```python
from build123d import *

# Parameters (mm, degrees)
IZIM1_R                     = 2.5
Y_KSEKLIK_EKSTR_ZYON1_DEPTH = 6
IZIM5_R                     = 0.246458924
IZIM7_R                     = 0.245


with BuildPart() as part:
    # Çizim1 → Yükseklik-Ekstrüzyon1 (new body)
    with BuildSketch(Plane(origin=(0, 0, 0), x_dir=(0, 0, -1), z_dir=(1, 0, 0))):
        Circle(IZIM1_R)
    extrude(amount=Y_KSEKLIK_EKSTR_ZYON1_DEPTH)

    # Süpür1: sweep along a path in Çizim4
    with BuildLine(Plane.XY) as s_p_r1_path:
        Line((0, 0), (-2.33257059, 0))
        ThreePointArc((-2.33257059, 0), (-2.732509931, -0.165660299), (-2.89817023, -0.56559964))
        Line((-2.89817023, -0.56559964), (-2.89817023, -8.872558098))
    # Çizim5 → Süpür1 (sweep)
    with BuildSketch(Plane(origin=(-2.89817023, -8.872558098, 0), x_dir=(-1, 0, 0), z_dir=(0, -1, 0))):
        with Locations((-0.000978554, 0)):
            Circle(IZIM5_R)
    sweep(path=s_p_r1_path.line)

    # Süpür2: sweep along a path in Çizim6
    with BuildLine(Plane.XY) as s_p_r2_path:
        Line((6, 0), (8.33, 0))
        ThreePointArc((8.33, 0), (8.931040764, -0.248959236), (9.18, -0.85))
        Line((9.18, -0.85), (9.18, -9.16))
    # Çizim7 → Süpür2 (sweep)
    with BuildSketch(Plane(origin=(9.18, -9.16, 0), x_dir=(-1, 0, 0), z_dir=(0, -1, 0))):
        with Locations((-0.002407495, 0)):
            Circle(IZIM7_R)
    sweep(path=s_p_r2_path.line)


solid = part.part
```
Geometry: final body of the model. Coordinates: model frame, mm. Round coordinates to 2 decimals unless told otherwise and drop trailing zeros. Write each loop counter-clockwise with the first axis right and the second up, starting at its lowest first coordinate (ties: lowest second). Pieces come first, ordered by that corner, then holes.
Item 1: Pin query (flat end, axial travel): P1, Ø2, axis at y = -3.5, z = 2, coming from the +X side. Return the tip coordinate at first contact, or that it passes through.
Item 2: Material intervals for L1, parallel to X at y = 1, z = 2.1; L2, parallel to Y at x = -0.5, z = 0; L3, parallel to Y at x = 3, z = 0.2, sorted ascending.
Item 3: Section query C-C (y = -3.5). Return loops of the section in (x, z) (3 decimals), plus the area to 3 significant figures.
Item 4: Section query D-D (x = -1). Return loops of the section in (y, z).
Item 5: Section query A-A (y = -2). Return loops of the section in (x, z) (3 decimals).
Item 6: Section query B-B (z = 0). Return loops of the section in (x, y), plus the area to 3 significant figures.
Completed:
1. P1: passes through
2. L1: x = 0 to 6
2. L2: y = -0.25 to 0.25
2. L3: y = -2.49 to 2.49
3. outline: circle Ø0.493 at (-2.897, 0); circle Ø0.49 at (9.182, 0)
3. area: 0.379 mm2
4. outline: circle Ø0.49 at (0, 0)
5. outline: circle Ø0.493 at (-2.897, 0); (0, -1.5) - (6, -1.5) - (6, 1.5) - (0, 1.5) - close; circle Ø0.49 at (9.182, 0)
6. outline: (-3.14, -8.87) - (-2.65, -8.87) - (-2.65, -0.57) arc R0.32 cw to (-2.33, -0.25) - (0, -0.25) - (0, -2.5) - (6, -2.5) - (6, -0.24) - (8.33, -0.24) arc R0.61 cw to (8.94, -0.85) - (8.94, -9.16) - (9.43, -9.16) - (9.43, -0.85) arc R1.1 ccw to (8.33, 0.25) - (6, 0.25) - (6, 2.5) - (0, 2.5) - (0, 0.25) - (-2.33, 0.25) arc R0.81 ccw to (-3.14, -0.57) - close
6. area: 41.6 mm2
